Work out the finished part from the listing and answer in its coordinate system (mm). Face numbers are marked on the shaded views. Coordinates: 2 decimals unless noted, no trailing zeros. Write each loop counter-clockwise with the first axis right and the second up, starting at its lowest first coordinate (ties: lowest second). Pieces come first, ordered by that corner, then holes. Notation, with made-up numbers: (58.5, 89.5) - (78.5, 89.5) arc R17 ccw to (78.5, 96.5) - close; hole circle Ø2 at (76.5, 62). An arc over 180 degrees is marked (long way). Use a Markdown table: item, result. Add a question column.
(1) The part is cut by section B-B, the plane y = -78.5. Give the vertices of the cut face in (x, z).
(2) Find the intervals of material crossed by line 1 (Z direction, x = 6, y = -60.5); line 2 (Y direction, x = 37, z = 24.5); line 3 (X direction, y = 23, z = 5), in increasing order. Write a range as from..to.
(3) Given pin 1 Ø12 at (y, z) = (40, 15.5) entering from -X, flat-ended and moving along its own axis, determine where the tip first touches the part or whether it passes through.
(4) The part is cut by section A-A, the plane x = 13. Give the vertices of the cut face in (y, z), then the cut area to 3 significant figures.
(5) For a pull along X with two mould halves and no side action, classify the marked faces 1 and 2 as released by +X, released by -X, zero draft, split by the parting line, or undercut.
(6) The part is cut by section C-C, the plane z = 9. Give the vertices of the cut face in (x, y), then the cut area to 3 significant figures.
from build123d import *

# Parameters (mm, degrees)
F0_W     = 400
F0_H     = 300
F1_DEPTH = 30
F2_SIZE  = 20
F3_SIZE  = 5
F4_T     = -3


with BuildPart() as f1:
    # F0 (on Top) → F1 (new body)
    with BuildSketch(Plane.XY):
        Rectangle(F0_W, F0_H)
    extrude(amount=F1_DEPTH)

    # F2
    f2_edges = [f1.edges().sort_by_distance(p)[0] for p in [
        (200, -150, 15),
        (200, 150, 15),
    ]]
    chamfer(f2_edges, length=F2_SIZE)

    # F3
    f3_edges = [f1.edges().sort_by_distance(p)[0] for p in [
        (-200, -150, 15),
        (-200, 150, 15),
    ]]
    chamfer(f3_edges, length=F3_SIZE)

    # F4
    f4_openings = [f1.faces().sort_by_distance(p)[0] for p in [
        (-200, 0, 15),
    ]]
    offset(amount=F4_T, openings=f4_openings)


solid = f1.part
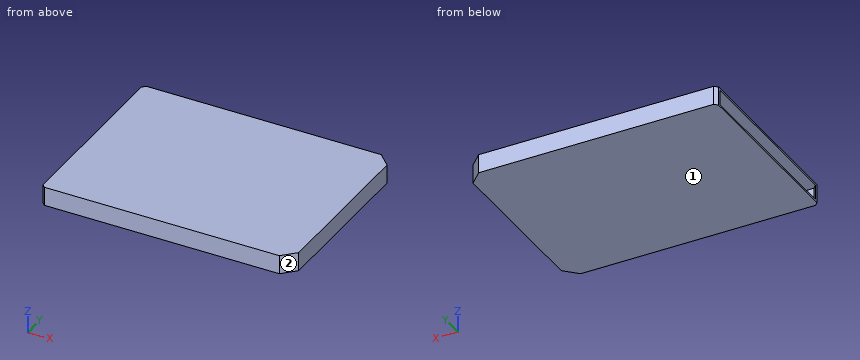
Model answer:
| question | item | result |
|---|---|---|
| 1 | outline | (-200, 0) - (200, 0) - (200, 30) - (-200, 30) - (-200, 27) - (197, 27) - (197, 3) - (-200, 3) - close |
| 2 | line 1 | 0..3, 27..30 |
| 2 | line 2 | -150..-147, 147..150 |
| 2 | line 3 | 197..200 |
| 3 | pin 1 | x = 197 |
| 4 | outline | (-150, 0) - (150, 0) - (150, 30) - (-150, 30) - close; hole (-147, 3) - (147, 3) - (147, 27) - (-147, 27) - close |
| 4 | area | 1,940 mm^2 |
| 5 | face 1 | zero draft |
| 5 | face 2 | released by +X |
| 6 | outline | (-200, -145) - (-195, -150) - (180, -150) - (200, -130) - (200, 130) - (180, 150) - (-195, 150) - (-200, 145) - (-200, 140.76) - (-193.76, 147) - (178.76, 147) - (197, 128.76) - (197, -128.76) - (178.76, -147) - (-193.76, -147) - (-200, -140.76) - close |
| 6 | area | 3,230 mm^2 |
